Autodesk Inventor part; units mm, degrees
ref_plane "Work Plane1" through (-153, 0, 0) normal (1, 0, 0) x (0, 1, 0)
ref_plane "XZ Plane" through (0, 0, 0) normal (0, 1, 0) x (-1, 0, 0)
ref_plane "XY Plane" through (0, 0, 0) normal (0, 0, 1) x (1, 0, 0)
sketch "Reinforcment" plane through (0, 0, 0) normal (0, 0, 1) x (1, 0, 0)
  line L0 (0, 0) -> (-150, 0)
  line L1 (-150, 0) -> (-150, 51.5)
  line L2 (-150, 51.5) -> (0, 50)
  line L3 (-154.0291, 0.0806) -> (-152.94, 54.5296)
  line L4 (-152.94, 54.5296) -> (0, 53.0001)
  line L5 (-150, 0) -> (-154.0291, 0.0806)
  line L6 (0, 50) -> (0, 53.0001)
  dimension "d1" = 50
  dimension "d2" = 51.5
  dimension "d3" = 3
revolve "Revolution1" add sketch "Reinforcment" angle 360 about axis through (0, 0, 0) along (-1, 0, 0)
sketch "Sketch2" plane through (0, 0, 0) normal (1, 0, 0) x (0, 0, -1)
  circle A0 centre (0, 0) radius 50
  line L0 (0, 50) -> (2, 50)
  line L1 (2, 50) -> (2, 41)
  line L2 (2, 41) -> (0, 41)
  line L3 (0, 50) -> (-2, 50)
  line L4 (-2, 50) -> (-2, 41)
  line L5 (-2, 41) -> (0, 41)
  line L6 (-43.3013, 25) -> (-42.3013, 26.7321)
  line L7 (-42.3013, 26.7321) -> (-34.507, 22.2321)
  line L8 (-34.507, 22.2321) -> (-35.507, 20.5)
  line L9 (-43.3013, 25) -> (-44.3013, 23.2679)
  line L10 (-44.3013, 23.2679) -> (-36.507, 18.7679)
  line L11 (-36.507, 18.7679) -> (-35.507, 20.5)
  line L12 (-43.3013, -25) -> (-44.3013, -23.2679)
  line L13 (-44.3013, -23.2679) -> (-36.507, -18.7679)
  line L14 (-36.507, -18.7679) -> (-35.507, -20.5)
  line L15 (-43.3013, -25) -> (-42.3013, -26.7321)
  line L16 (-42.3013, -26.7321) -> (-34.507, -22.2321)
  line L17 (-34.507, -22.2321) -> (-35.507, -20.5)
  line L18 (0, -50) -> (-2, -50)
  line L19 (-2, -50) -> (-2, -41)
  line L20 (-2, -41) -> (0, -41)
  line L21 (0, -50) -> (2, -50)
  line L22 (2, -50) -> (2, -41)
  line L23 (2, -41) -> (0, -41)
  line L24 (43.3013, -25) -> (42.3013, -26.7321)
  line L25 (42.3013, -26.7321) -> (34.507, -22.2321)
  line L26 (34.507, -22.2321) -> (35.507, -20.5)
  line L27 (43.3013, -25) -> (44.3013, -23.2679)
  line L28 (44.3013, -23.2679) -> (36.507, -18.7679)
  line L29 (36.507, -18.7679) -> (35.507, -20.5)
  line L30 (43.3013, 25) -> (44.3013, 23.2679)
  line L31 (44.3013, 23.2679) -> (36.507, 18.7679)
  line L32 (36.507, 18.7679) -> (35.507, 20.5)
  line L33 (43.3013, 25) -> (42.3013, 26.7321)
  line L34 (42.3013, 26.7321) -> (34.507, 22.2321)
  line L35 (34.507, 22.2321) -> (35.507, 20.5)
  point P0 (44.2666, 23.2479)
  point P1 (42.2666, 26.712)
  point P2 (42.2666, -26.712)
  point P3 (44.2666, -23.2479)
  point P4 (0, -41)
  point P5 (-2, -49.96)
  point P6 (2, -49.96)
  point P7 (-44.2666, -23.2479)
  point P8 (-42.2666, -26.712)
  point P9 (-42.2666, 26.712)
  point P10 (-44.2666, 23.2479)
  point P11 (2, 49.96)
  point P12 (-2, 49.96)
  dimension "d5" = 2
  dimension "d6" = 9
  dimension "d7" = 2
  dimension "d10" = 360
extrude "Extrusion1" add sketch "Sketch2" against normal up to next contours L31 L32 L35 L34 A0 | A0 L25 L26 L29 L28 | L1 L2 L5 L4 A0 | A0 L19 L20 L23 L22 | L7 L8 L11 L10 A0 | A0 L13 L14 L17 L16
sketch "Sketch3" plane through (0, 0, 0) normal (1, 0, 0) x (0, 0, -1)
  circle A0 centre (0, 0) radius 53.8081
  circle A1 centre (0, 0) radius 50
  line L0 (0, 50) -> (1.5, 50)
  line L1 (1.5, 50) -> (1.5, 46)
  line L2 (1.5, 46) -> (0, 46)
  line L3 (0, 50) -> (-1.5, 50)
  line L4 (-1.5, 50) -> (-1.5, 46)
  line L5 (-1.5, 46) -> (0, 46)
  line L6 (-43.3013, 25) -> (-42.5513, 26.299)
  line L7 (-42.5513, 26.299) -> (-39.0872, 24.299)
  line L8 (-39.0872, 24.299) -> (-39.8372, 23)
  line L9 (-43.3013, 25) -> (-44.0513, 23.701)
  line L10 (-44.0513, 23.701) -> (-40.5872, 21.701)
  line L11 (-40.5872, 21.701) -> (-39.8372, 23)
  line L12 (-43.3013, -25) -> (-44.0513, -23.701)
  line L13 (-44.0513, -23.701) -> (-40.5872, -21.701)
  line L14 (-40.5872, -21.701) -> (-39.8372, -23)
  line L15 (-43.3013, -25) -> (-42.5513, -26.299)
  line L16 (-42.5513, -26.299) -> (-39.0872, -24.299)
  line L17 (-39.0872, -24.299) -> (-39.8372, -23)
  line L18 (0, -50) -> (-1.5, -50)
  line L19 (-1.5, -50) -> (-1.5, -46)
  line L20 (-1.5, -46) -> (0, -46)
  line L21 (0, -50) -> (1.5, -50)
  line L22 (1.5, -50) -> (1.5, -46)
  line L23 (1.5, -46) -> (0, -46)
  line L24 (43.3013, -25) -> (42.5513, -26.299)
  line L25 (42.5513, -26.299) -> (39.0872, -24.299)
  line L26 (39.0872, -24.299) -> (39.8372, -23)
  line L27 (43.3013, -25) -> (44.0513, -23.701)
  line L28 (44.0513, -23.701) -> (40.5872, -21.701)
  line L29 (40.5872, -21.701) -> (39.8372, -23)
  line L30 (43.3013, 25) -> (44.0513, 23.701)
  line L31 (44.0513, 23.701) -> (40.5872, 21.701)
  line L32 (40.5872, 21.701) -> (39.8372, 23)
  line L33 (43.3013, 25) -> (42.5513, 26.299)
  line L34 (42.5513, 26.299) -> (39.0872, 24.299)
  line L35 (39.0872, 24.299) -> (39.8372, 23)
  point P0 (-42.5318, 26.2878)
  point P1 (-44.0318, 23.6897)
  point P2 (-44.0318, -23.6897)
  point P3 (-42.5318, -26.2878)
  point P4 (0, -46)
  point P5 (-1.5, -49.9775)
  point P6 (1.5, -49.9775)
  point P7 (42.5318, -26.2878)
  point P8 (44.0318, -23.6897)
  point P9 (44.0318, 23.6897)
  point P10 (42.5318, 26.2878)
  point P11 (1.5, 49.9775)
  point P12 (-1.5, 49.9775)
  dimension "d32" = 1.5
  dimension "d33" = 4
  dimension "d34" = 1.5
  dimension "d37" = 360
extrude "Extrusion2" cut sketch "Sketch3" against normal blind 20 contours L31 L32 L35 L34 A1 | A1 L25 L26 L29 L28 | L1 L2 L5 L4 A1 | A1 L19 L20 L23 L22 | L7 L8 L11 L10 A1 | A1 L13 L14 L17 L16
ref_plane "Work Plane1" through (-153, 0, 0) normal (1, 0, 0) x (0, 1, 0)
sketch "Sketch5" plane through (-153, 0, 0) normal (1, 0, 0) x (0, 1, 0)
  circle A0 centre (0, 0) radius 51.5
  circle A1 centre (0, 0) radius 49.875
  dimension "d28" = 103
  dimension "d29" = 99.75
extrude "Extrusion4" add sketch "Sketch5" against normal blind 60
equation "\"BendRadius\" = Thickness"
equation "\"BendReliefWidth\" = Thickness"
equation "\"BendReliefDepth\" = 0.5 * Thickness"
equation "\"CornerReliefSize\" = 4 * Thickness"
equation "\"MinimumRemnant\" = 2 * Thickness"
equation "\"TransitionRadius\" = BendRadius"
equation "\"JacobiRadiusSize\" = BendRadius"
equation "\"GapSize\" = Thickness"
properties part number "Nosecone(finale)"
Source: CAD feature listing. Evaluate the final solid. Frame: model axes, mm. A direction names the side the tool comes from. Coordinates: 2 decimals unless noted, no trailing zeros. Loops run counter-clockwise (first coordinate to the right, second up) from the corner with the lowest first, then second, coordinate; pieces in that order, holes last. Notation, with made-up numbers: M 33.25,-39.75 L 79.25,-39.75 A20 cw 79.25,-21.75 Z; hole C 38.5,64.5 d4. An arc over 180 degrees is marked long. Use a Markdown table: item, result. Add a question column.
Q1. Section query B-B, the plane x = -200. Return loops of the section in (y, z) (3 decimals).
Q2. Section query A-A, the plane x = -84.5. Return loops of the section in (y, z) (3 decimals), and give its area (3 significant figures).
Q3. Material intervals for L1, parallel to Y at x = -196, z = 0 (3 decimals); L2, parallel to Y at x = -51, z = -1, sorted ascending.
Q4. Draft query along Z for faces 4 (the flat face through (0, -22, 38)), 5 (the flat face through (-74, 46, 2)), 6 (the flat face through (-73.95, 21.04, 40.44)). Return one class per face: pulls with the +Z half, pulls with the -Z half, needs draft (parallel to the pull), parting line crosses it, or undercut.
Q5. First-contact query: pin 1 (3 mm diameter, centred on x = -15, y = -49, fed in from -Z); pin 2 (2 mm diameter, centred on x = -98, y = 38, fed in from +Z); pin 3 (2 mm diameter, centred on x = -6, y = -47.5, fed in from +Z). Flat tips, straight axial feed; report the tip coordinate or a pass-through.
Q6. Access query for faces 1 (the flat face through (-20, -24, -42)), 2 (the cylindrical face through (-74, -50, 0)), 3 (the flat face through (0, 22, 38)). Directions: +Z, -Z, +X, -X, +Y, -Y. A direction counts if a zero-diameter tool reaches every point of the face in a straight line with its end or side. Return the directions, or none.
Result:
| question | item | result |
|---|---|---|
| 1 | outline | C 0,0 d103; hole C 0,0 d99.75 |
| 2 | outline | C 0,0 d107.69; M -49.96,-2 L -41,-2 L -41,2 L -49.96,2 A50 ccw Z; M -26.712,-42.267 A50 ccw -23.248,-44.267 L -18.768,-36.507 L -22.232,-34.507 Z; M -26.712,42.267 L -22.232,34.507 L -18.768,36.507 L -23.248,44.267 A50 ccw Z; M 18.768,-36.507 L 23.248,-44.267 A50 ccw 26.712,-42.267 L 22.232,-34.507 Z; M 18.768,36.507 L 22.232,34.507 L 26.712,42.267 A50 ccw 23.248,44.267 Z; M 41,-2 L 49.96,-2 A50 ccw 49.96,2 L 41,2 Z; hole C 0,0 d101.69 |
| 2 | area | 1,200 mm2 |
| 3 | L1 | y = -51.5 to -49.875, 49.875 to 51.5 |
| 3 | L2 | y = -53.5 to -50.5, -49.99 to -41, 41 to 49.99, 50.5 to 53.5 |
| 4 | face 4 | needs draft |
| 4 | face 5 | undercut |
| 4 | face 6 | undercut |
| 5 | pin 1 | stops at z = -23.85 |
| 5 | pin 2 | stops at z = 39.3 |
| 5 | pin 3 | stops at z = 25.56 |
| 6 | face 1 | +X |
| 6 | face 2 | none |
| 6 | face 3 | +Z, -Z, +X, +Y, -Y |
